from build123d import *

# Parameters (mm, degrees)
F0_R            = 30
F0_R_2          = 10
F1_DEPTH        = 70
F2_R            = 10
F3_DEPTH        = 130
F3_DEPTH_BACK   = 70
F5_DEPTH        = 70
F5_COPIES_COUNT = 4


# Not quite as in the source:
# - a pattern or mirror of a feature is missing from the dataset's text; its kind, count and spacing are read off the source's solid


with BuildPart() as f1:
    # F0 (on Top) → F1 (new body)
    with BuildSketch(Plane.XY):
        Circle(F0_R)
        Circle(F0_R_2, mode=Mode.SUBTRACT)
    extrude(amount=F1_DEPTH)

    # F2 (on face) → F3 (join, two sides)
    with BuildSketch(Plane.XY.offset(70)) as f3_sk:
        Circle(F2_R)
    extrude(amount=F3_DEPTH)
    extrude(f3_sk.sketch, amount=-F3_DEPTH_BACK)

    # F4 (on face) → F5 (cut, through all)
    with BuildSketch(Plane.XY.offset(70)):
        with BuildLine():
            ThreePointArc((3.4286095737, -9.3938616336), (0, -10), (-3.4286095737, -9.3938616336))
            Line((-3.4286095737, -9.3938616336), (-10.9373596855, -27.9351778786))
            ThreePointArc((-10.9373596855, -27.9351778786), (0, -30), (10.9373596855, -27.9351778786))
            Line((10.9373596855, -27.9351778786), (3.4286095737, -9.3938616336))
        make_face()
    f5 = extrude(amount=-F5_DEPTH, mode=Mode.SUBTRACT)

    # F5_copies: F5 ×4 about axis
    f5_copies_axis = Axis((0, 0, 0), (0, 0, 1))
    for i in range(1, F5_COPIES_COUNT):
        add(f5.rotate(f5_copies_axis, i * 360 / F5_COPIES_COUNT), mode=Mode.SUBTRACT)


solid = f1.part
Design review of the part built by this model. Coordinates are the model's own, in mm. A direction names the side the tool comes from. Give positions to 0.01 mm unless a question says otherwise; leave off trailing zeros. Loops run counter-clockwise (first coordinate to the right, second up) from the corner with the lowest first, then second, coordinate; pieces in that order, holes last. Notation, with made-up numbers: (29.5, 23) -> (67.5, 23) arc R15 ccw to (67.5, 50) -> close; hole circle Ø4 at (17, 13.5). An arc over 180 degrees is marked (long way). One line per question, with ' | ' between items. Start each with the question number.
(1) We need section B-B (x = -18). State the section outline as (y, z) points, and give its area (3 significant figures).
(2) We need section C-C (z = 32.5). State the section outline as (x, y) points.
(3) For faces 4 (the face through (7.236, -18.794, 35.49)), 5 (the face through (7.13, 18.53, 35.49)), 6 (the face through (-18.53, 7.13, 35.49)), 7 (the face through (-16, 16, 70)), 8 (the face through (18.53, -7.13, 35.49)), list the 3-axis set-ups (+Z, -Z, +X, -X, +Y, -Y) from which the entire face can be reached by the end or side of a thin tool; tool diameter is ignored.
(4) For line 1 (X direction, y = 22.5, z = 40.5); line 2 (Z direction, x = -19, y = 22); line 3 (X direction, y = 0.5, z = 192), list the stretches that pass through material, from the lowest coordinate up.
(5) We need section A-A (y = 21). State the section outline as (x, z) points.
(6) We need section D-D (x = 7.5). State the section outline as (y, z) points.
(7) Draft analysis for pull direction Y (two halves, no side actions). For faces 1 (the face through (-18.794, -7.236, 35.49)), 2 (the face through (0, 0, 200)), 3 (the face through (-7.236, 18.794, 35.49)), state which applies: +Y half, -Y half, draft (parallel to the pull), parting line (faces both ways), or undercut.
(8) Insertion check: P1, Ø5, axis at x = 13, y = -10, coming from the +Z side; P2, Ø5, axis at x = -7, z = 36.5, coming from the +Y side; P3, Ø1, axis at x = 4, z = 140, coming from the +Y side. Each pin has a flat end and moves straight along its axis. Give the tip position at first contact, or say it passes through.
The answers:
1) outline: (-24, 0) -> (-6.91, 0) -> (-6.91, 70) -> (-24, 70) -> close; (6.91, 0) -> (24, 0) -> (24, 70) -> (6.91, 70) -> close | area: 2,390 mm^2
2) outline: (-27.94, -10.94) arc R30 ccw to (-10.94, -27.94) -> (-3.43, -9.39) arc R10 ccw to (3.43, -9.39) -> (10.94, -27.94) arc R30 ccw to (27.94, -10.94) -> (9.39, -3.43) arc R10 ccw to (9.39, 3.43) -> (27.94, 10.94) arc R30 ccw to (10.94, 27.94) -> (3.43, 9.39) arc R10 ccw to (-3.43, 9.39) -> (-10.94, 27.94) arc R30 ccw to (-27.94, 10.94) -> (-9.39, 3.43) arc R10 ccw to (-9.39, -3.43) -> close
3) face 4: +Z, -Z, -Y | face 5: +Z, -Z, +Y | face 6: +Z, -Z, -X | face 7: +Z, -X, +Y | face 8: +Z, -Z, +X
4) line 1: x = -19.84 to -8.74, 8.74 to 19.84 | line 2: z = 0 to 70 | line 3: x = -9.99 to 9.99
5) outline: (-21.42, 0) -> (-8.13, 0) -> (-8.13, 70) -> (-21.42, 70) -> close; (8.13, 0) -> (21.42, 0) -> (21.42, 70) -> (8.13, 70) -> close
6) outline: (-19.45, 0) -> (19.45, 0) -> (19.45, 70) -> (6.61, 70) -> (6.61, 200) -> (-6.61, 200) -> (-6.61, 70) -> (-19.45, 70) -> close
7) face 1: undercut | face 2: draft | face 3: +Y half
8) P1: stops at z = 70 | P2: stops at y = 24.39 | P3: stops at y = 9.37
